```python
from build123d import *

# Parameters (mm, degrees)
BOSS_EXTRUDE1_DEPTH = 55
FILLET1_R           = 4
FILLET2_R           = 1.5
SKETCH2_R           = 23
CUT_EXTRUDE1_DEPTH  = 102.118742081
SCALE1_SCALE        = 2.3


with BuildPart() as part:
    # Sketch1 → Boss-Extrude1 (new body)
    with BuildSketch(Plane.XY):
        Polygon((9, 0), (51, 0), (51, 9), (60, 9), (60, 51), (51, 51), (51, 60), (9, 60), (9, 51), (0, 51), (0, 9), (9, 9), align=None)
    extrude(amount=BOSS_EXTRUDE1_DEPTH)

    # Fillet1
    fillet1_edges = [part.edges().sort_by_distance(p)[0] for p in [
        (9, 9, 27.5),
        (9, 51, 27.5),
        (51, 51, 27.5),
        (51, 9, 27.5),
    ]]
    fillet(fillet1_edges, radius=FILLET1_R)

    # Fillet2
    fillet2_edges = [part.edges().sort_by_distance(p)[0] for p in [
        (51, 0, 27.5),
        (9, 0, 27.5),
        (0, 9, 27.5),
        (0, 51, 27.5),
        (9, 60, 27.5),
        (51, 60, 27.5),
        (60, 51, 27.5),
        (60, 9, 27.5),
    ]]
    fillet(fillet2_edges, radius=FILLET2_R)

    # Sketch2 → Cut-Extrude1 (cut, through all)
    with BuildSketch(Plane.XY.offset(55)):
        with Locations((30, 30)):
            Circle(SKETCH2_R)
    extrude(amount=-CUT_EXTRUDE1_DEPTH, mode=Mode.SUBTRACT)


with BuildPart() as part_1:
    # Scale1: scaled about (30, 30, 27.5)
    add(part.part.scale(SCALE1_SCALE).moved(Location((-39, -39, -35.75))))


solid = part_1.part
```
Work out the finished part from the listing and answer in its coordinate system (mm). A direction names the side the tool comes from. Coordinates: 2 decimals unless noted, no trailing zeros. Write each loop counter-clockwise with the first axis right and the second up, starting at its lowest first coordinate (ties: lowest second). Pieces come first, ordered by that corner, then holes.
Q1. Find the intervals of material crossed by line 1 (Y direction, x = 30, z = 46); line 2 (Y direction, x = 14.5, z = 0); line 3 (X direction, y = -1, z = 76), in increasing order.
Q2. A cutting plane is placed at B-B, the plane z = 35. Give the vertices of the cut face in (x, y).
Q3. Each of these flat-tipped pins is pushed along its axis until it touches: pin 1 Ø4 at (x, z) = (-30.5, 17) entering from +Y; pin 2 Ø9 at (y, z) = (90, 10) entering from +X; pin 3 Ø2.5 at (y, z) = (91.5, 47.5) entering from -X; pin 4 Ø12 at (x, y) = (70, 2.5) entering from -Z. Where does it stop, or does it pass through?
Q4. Determine the mould class of faces 1 (the face through (80.92, -21.07, 28.39)), 2 (the face through (18.53, -21.64, 28.39)), 3 (the face through (-31, 78.3, 27)) for opening direction Y: released by +Y, released by -Y, zero draft, split by the parting line, or undercut.
Q5. Which of the six approach directions +Z, -Z, +X, -X, +Y, -Y give full straight-line access (tool end or side, diameter ignored) to faces 4 (the face through (78.3, -32, 27)), 5 (the face through (-32, -18.3, 27)), 6 (the face through (-18.3, 92, 27))?
Q6. A cutting plane is placed at C-C, the plane x = 33. Give the vertices of the cut face in (y, z).
Q7. A cutting plane is placed at A-A, the plane y = 30. Give the vertices of the cut face in (x, z).
Findings below:
1. line 1: y = -39 to -22.9, 82.9 to 99
1. line 2: y = -39 to -20.58, 80.58 to 99
1. line 3: x = -39 to -12.87, 72.87 to 99
2. outline: (-39, -14.85) arc R3.45 ccw to (-35.55, -18.3) - (-27.5, -18.3) arc R9.2 cw to (-18.3, -27.5) - (-18.3, -35.55) arc R3.45 ccw to (-14.85, -39) - (74.85, -39) arc R3.45 ccw to (78.3, -35.55) - (78.3, -27.5) arc R9.2 cw to (87.5, -18.3) - (95.55, -18.3) arc R3.45 ccw to (99, -14.85) - (99, 74.85) arc R3.45 ccw to (95.55, 78.3) - (87.5, 78.3) arc R9.2 cw to (78.3, 87.5) - (78.3, 95.55) arc R3.45 ccw to (74.85, 99) - (-14.85, 99) arc R3.45 ccw to (-18.3, 95.55) - (-18.3, 87.5) arc R9.2 cw to (-27.5, 78.3) - (-35.55, 78.3) arc R3.45 ccw to (-39, 74.85) - close; hole circle Ø105.8 at (30, 30)
3. pin 1: stops at y = 78.3
3. pin 2: stops at x = 78.52
3. pin 3: stops at x = -18.3
3. pin 4: stops at z = -35.75
4. face 1: released by -Y
4. face 2: undercut
4. face 3: released by +Y
5. face 4: +Z, -Z, +X, -Y
5. face 5: +Z, -Z, -X, -Y
5. face 6: +Z, -Z, -X, +Y
6. outline: (-39, -35.75) - (-22.81, -35.75) - (-22.81, 90.75) - (-39, 90.75) - close; (82.81, -35.75) - (99, -35.75) - (99, 90.75) - (82.81, 90.75) - close
7. outline: (-39, -35.75) - (-22.9, -35.75) - (-22.9, 90.75) - (-39, 90.75) - close; (82.9, -35.75) - (99, -35.75) - (99, 90.75) - (82.9, 90.75) - close
